from build123d import *

# Parameters (mm, degrees)
F0_R     = 6.5
F1_DEPTH = 33
F0_R_2   = 18.75
F2_DEPTH = 28.5
F3_R     = 6.5
F4_DEPTH = 34
F5_R     = 1.5875
F6_DEPTH = 42


with BuildPart() as f1:
    # F0 (on Top) → F1 (new body)
    with BuildSketch(Plane.XY):
        Circle(F0_R)
    extrude(amount=F1_DEPTH)

    # F0 (on Top) → F2 (join, symmetric)
    with BuildSketch(Plane.XY):
        Circle(F0_R_2)
        Circle(F0_R, mode=Mode.SUBTRACT)
    extrude(amount=F2_DEPTH, both=True)

    # F3 (on Top) → F4 (join)
    with BuildSketch(Plane.XY):
        Circle(F3_R)
    extrude(amount=-F4_DEPTH)

    # F5 (on Top) → F6 (join)
    with BuildSketch(Plane.XY):
        Circle(F5_R)
    extrude(amount=F6_DEPTH)


solid = f1.part
Build history of the part. All positions in model axes, mm. A direction names the side the tool comes from. Coordinates: 2 decimals unless noted, no trailing zeros. Order: outer loops, then holes, each group sorted by start corner. A loop starts at its lowest first (then second) coordinate and runs counter-clockwise, first axis right, second up. Notation, with made-up numbers: (-31.75, 76.5) -> (-2.75, 76.5) arc R13 cw to (-2.75, 100.5) -> close; hole circle Ø4 at (-22, 78.5). An arc over 180 degrees is marked (long way). One line per item, written item: value.
(1) Slice it at D-D, the plane y = -4.5. List the corners of the cut face in (x, z), plus the area to 3 significant figures.
Checked values:
outline: (-18.2, -28.5) -> (-4.69, -28.5) -> (-4.69, -34) -> (4.69, -34) -> (4.69, -28.5) -> (18.2, -28.5) -> (18.2, 28.5) -> (4.69, 28.5) -> (4.69, 33) -> (-4.69, 33) -> (-4.69, 28.5) -> (-18.2, 28.5) -> close
area: 2,170 mm2
(2) Tool access for faces 1 (the cylindrical face through (-5.158, -3.955, -31.212)), 2 (the cylindrical face through (-2.44, 18.59, 0.4)), 3 (the flat face through (1.4, -1.4, 33)): list every direction of +Z, -Z, +X, -X, +Y, -Y with a clear straight run to the whole face (end or side of a thin tool).
Checked values:
face 1: -Z
face 2: +Z, -Z
face 3: +Z
(3) Slice it at C-C, the plane z = 29.5. List the corners of the cut face in (x, y), plus the area to 3 significant figures.
Checked values:
outline: circle Ø13 at (0, 0)
area: 133 mm2
(4) Probe line 1 (Z direction, x = -10, y = 10); line 2 (Z direction, x = -3, y = 0); line 3 (Y direction, x = -3, z = -22). List the from-to ranges inside material, lowest first. Write a range as [from, to].
Checked values:
line 1: [-28.5, 28.5]
line 2: [-34, 33]
line 3: [-18.51, 18.51]
(5) Slice it at A-A, the plane x = 0. List the corners of the cut face in (y, z).
Checked values:
outline: (-18.75, -28.5) -> (-6.5, -28.5) -> (-6.5, -34) -> (6.5, -34) -> (6.5, -28.5) -> (18.75, -28.5) -> (18.75, 28.5) -> (6.5, 28.5) -> (6.5, 33) -> (1.59, 33) -> (1.59, 42) -> (-1.59, 42) -> (-1.59, 33) -> (-6.5, 33) -> (-6.5, 28.5) -> (-18.75, 28.5) -> close
(6) Drop flat-ended pins along their axis: pin 1 Ø3 at (y, z) = (13, 23) entering from -X; pin 2 Ø1.5 at (y, z) = (1.5, -22.5) entering from -X (3 decimals); pin 3 Ø1 at (x, y) = (14.5, -14.5) entering from -Z; pin 4 Ø6.5 at (x, y) = (1.5, -1) entering from +Z. Give the stop position or say it passes through.
Checked values:
pin 1: x = -14.81
pin 2: x = -18.735
pin 3: through
pin 4: z = 42
